```python
from build123d import *

# Parameters (mm, degrees)
F0_W          = 19.9
F0_H          = 10.7
F1_DEPTH      = 3.075
F1_DEPTH_BACK = 3.075
F2_W          = 1.5
F2_H          = 4
F3_DEPTH      = 1
F4_R          = 0.5
F6_DEPTH      = 4
F7_W          = 10.5
F7_H          = 0.7
F7_W_2        = 3.5
F7_H_2        = 0.5
F7_W_3        = 6.9
F7_R          = 1.5
F8_DEPTH      = 25
F9_SIZE       = 0.69999
F10_SIZE      = 0.49999


# Not quite as in the source:
# - a fillet or chamfer is up to 0.001 mm smaller than in the source, because OpenCascade refuses the exact size


with BuildPart() as f1:
    # F0 (on Top) → F1 (new body, two sides)
    with BuildSketch(Plane.XY) as f1_sk:
        Rectangle(F0_W, F0_H)
    extrude(amount=F1_DEPTH)
    extrude(f1_sk.sketch, amount=-F1_DEPTH_BACK)

    # F2 (on face) → F3 (join)
    with BuildSketch(Plane(origin=(0, 5.35, 0), x_dir=(-1, 0, 0), z_dir=(0, 1, 0))):
        with Locations((-3.2, 0)):
            Rectangle(F2_W, F2_H)
    extrude(amount=F3_DEPTH)

    # F4
    f4_edges = [f1.edges().sort_by_distance(p)[0] for p in [
        (2.45, 6.35, 0),
        (3.95, 6.35, 0),
    ]]
    fillet(f4_edges, radius=F4_R)

    # F5 (on face) → F6 (join)
    with BuildSketch(Plane(origin=(0, 0, -2), x_dir=(1, 0, 0), z_dir=(0, 0, -1))):
        with BuildLine():
            Line((6.75, -6.35), (6.75, -5.35))
            Line((6.75, -5.35), (6.5, -5.35))
            Line((6.5, -5.35), (6.5, -6.1638856134))
            Line((6.5, -6.1638856134), (-9.95, -11.089035314))
            Line((-9.95, -11.089035314), (-10.021705391, -11.110503994))
            Line((-10.021705391, -11.110503994), (-9.95, -11.35))
            Line((-9.95, -11.35), (-9.7212332774, -12.1140808536))
            ThreePointArc((-9.7212332774, -12.1140808536), (-6.8616282462, -15.4358597688), (-6.297976785, -11.08915376))
            Line((-6.297976785, -11.08915376), (-6.5267435076, -10.3250729065))
            Line((-6.5267435076, -10.3250729065), (6.75, -6.35))
        make_face()
    extrude(amount=-F6_DEPTH)

    # F7 (on face) → F8 (cut)
    with BuildSketch(Plane(origin=(0, 0, -3.075), x_dir=(1, 0, 0), z_dir=(0, 0, -1))):
        with Locations((-4.7, -5)):
            Rectangle(F7_W, F7_H)
        with Locations((-8.2, 5.1)):
            Rectangle(F7_W_2, F7_H_2)
        with Locations((8.2, 5.1)):
            Rectangle(F7_W_2, F7_H_2)
        with Locations((0, 5.1)):
            Rectangle(F7_W_3, F7_H_2)
        with Locations((4.95, 2.35)):
            Circle(F7_R)
        with Locations((-4.95, 2.35)):
            Circle(F7_R)
    extrude(amount=-F8_DEPTH, mode=Mode.SUBTRACT)

    # F9 (size 0.7 in the source; OpenCascade refuses exactly that, so slightly less here)
    f9_edges = [f1.edges().sort_by_distance(p)[0] for p in [
        (0.55, 4.65, 0),
    ]]
    chamfer(f9_edges, length=F9_SIZE)

    # F10 (size 0.5 in the source; OpenCascade refuses exactly that, so slightly less here)
    f10_edges = [f1.edges().sort_by_distance(p)[0] for p in [
        (6.45, -4.85, 0),
        (3.45, -4.85, 0),
        (-3.45, -4.85, 0),
        (-6.45, -4.85, 0),
    ]]
    chamfer(f10_edges, length=F10_SIZE)


solid = f1.part
```
Input: part model. Units: mm. Frame: model coordinates. A direction names the side the tool comes from. Round coordinates to 2 decimals unless told otherwise and drop trailing zeros. Write each loop counter-clockwise with the first axis right and the second up, starting at its lowest first coordinate (ties: lowest second). Pieces come first, ordered by that corner, then holes. Notation, with made-up numbers: M 75.25,-33.75 L 107.25,-33.75 A25 ccw 107.25,-5.75 Z; hole C 69,53 d4. An arc over 180 degrees is marked long. Write each question's results on one line, items separated by ' | '.
Q1. Pin query (flat end, axial travel): P1, Ø3, axis at x = -3.5, z = -1, coming from the +Y side; P2, Ø1.8, axis at y = -1.5, z = 1, coming from the -X side; P3, Ø2.5, axis at x = -4.95, y = -2.35, coming from the -Z side; P4, Ø3, axis at x = 1, z = 1, coming from the -Y side. Return the tip coordinate at first contact, or that it passes through.
Results:
P1: stops at y = 9.87 | P2: stops at x = -9.95 | P3: passes through | P4: stops at y = -4.85
Q2. Section query A-A (y = -2.35). Return loops of the section in (x, z) (3 decimals), and give its area (3 significant figures).
Results:
outline: M -9.95,-3.075 L -6.45,-3.075 L -6.45,3.075 L -9.95,3.075 Z; M -3.45,-3.075 L 3.45,-3.075 L 3.45,3.075 L -3.45,3.075 Z; M 6.45,-3.075 L 9.95,-3.075 L 9.95,3.075 L 6.45,3.075 Z | area: 85.5 mm^2
Q3. Line query: line 1 along X through (y, z) = (-2.25, 0); line 2 along Y through (x, z) = (5.5, 0.75); line 3 along Y through (x, z) = (-4.95, -0.25). Output: solid intervals per line, ascending.
Results:
line 1: x = -9.95 to -6.45, -3.45 to 3.45, 6.45 to 9.95 | line 2: y = -5.35 to -3.75, -0.95 to 5.35, 6.46 to 6.72 | line 3: y = -5.35 to -3.85, -0.85 to 4.65, 9.59 to 9.85
Q4. Draft query along Y for faces 1 (the face through (3, 6, -2)), 2 (the face through (6.5, 6, 0)), 3 (the face through (-8, -4.85, 0)), 4 (the face through (-6.936, 15.457, -0.028)). Return one class per face: released by +Y, released by -Y, zero draft, split by the parting line, or undercut.
Results:
face 1: zero draft | face 2: undercut | face 3: released by -Y | face 4: undercut
Q5. Section query B-B (z = -2.5). State how many separate pieces and enclosed holes the cut face has, and give its area (3 significant figures).
Results:
separate pieces: 1 | enclosed holes: 2 | area: 185 mm^2
Q6. Access query for faces 5 (the face through (-7, 12, -2)), 6 (the face through (3, 6, 2)), 7 (the face through (-9.95, 0, 0)), 8 (the face through (-5, 4.65, 0)). Directions: +Z, -Z, +X, -X, +Y, -Y. A direction counts if a zero-diameter tool reaches every point of the face in a straight line with its end or side. Return the directions, or none.
Results:
face 5: -Z, +X, -X, +Y | face 6: +Z, +X, -X, +Y | face 7: +Z, -Z, -X, -Y | face 8: +Z, -Z, -X
Q7. Section query D-D (x = -1.75). Return loops of the section in (y, z) (3 decimals).
Results:
outline: M -4.85,-3.075 L 4.65,-3.075 L 4.65,3.075 L -4.85,3.075 Z; M 8.634,-2 L 8.895,-2 L 8.895,2 L 8.634,2 Z
Q8. Section query C-C (x = 5.25). Return loops of the section in (y, z) (3 decimals), and give its area (3 significant figures).
Results:
outline: M -5.35,-3.075 L -3.82,-3.075 L -3.82,3.075 L -5.35,3.075 Z; M -0.88,-3.075 L 5.35,-3.075 L 5.35,3.075 L -0.88,3.075 Z; M 6.538,-2 L 6.799,-2 L 6.799,2 L 6.538,2 Z | area: 48.8 mm^2
